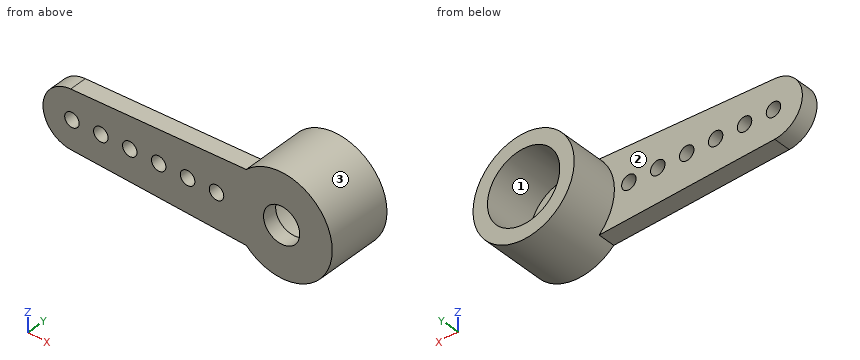
from build123d import *

# Parameters (mm, degrees)
SKETCH_1_R          = 0.5
EXTRUDE_1_DEPTH     = 1.2
SKETCH_1_3_R        = 3.5
SKETCH_1_3_R_2      = 2.5
EXTRUDE_2_DEPTH     = 4.5
SKETCH_1_4_R        = 2.5
EXTRUDE_3_DEPTH     = 1
SKETCH_3_R          = 1.25
CUT_EXTRUDE_1_DEPTH = 1


with BuildPart() as part:
    # 草图1 → 凸台-拉伸1 (new body)
    with BuildSketch(Plane(origin=(0, 0, 0), x_dir=(1, 0, 0), z_dir=(0, 1, 0))):
        with BuildLine():
            Line((4.682566803, 2.501585477), (-7.452442074, 1.998282013))
            ThreePointArc((-7.452442074, 1.998282013), (-9.369562674, 0), (-7.452442074, -1.998282013))
            Line((-7.452442074, -1.998282013), (4.682566803, -2.501585477))
            ThreePointArc((4.682566803, -2.501585477), (3.630437326, 0), (4.682566803, 2.501585477))
        make_face()
        with Locations((-7.369562674, 0)):
            Circle(SKETCH_1_R, mode=Mode.SUBTRACT)
        with Locations((-5.369562674, 0)):
            Circle(SKETCH_1_R, mode=Mode.SUBTRACT)
        with Locations((-3.369562674, 0)):
            Circle(SKETCH_1_R, mode=Mode.SUBTRACT)
        with Locations((-1.369562674, 0)):
            Circle(SKETCH_1_R, mode=Mode.SUBTRACT)
        with Locations((0.630437326, 0)):
            Circle(SKETCH_1_R, mode=Mode.SUBTRACT)
        with Locations((2.630437326, 0)):
            Circle(SKETCH_1_R, mode=Mode.SUBTRACT)
    extrude(amount=EXTRUDE_1_DEPTH)

    # 草图1<3> → 凸台-拉伸2 (add)
    with BuildSketch(Plane(origin=(0, 0, 0), x_dir=(1, 0, 0), z_dir=(0, 1, 0))):
        with Locations((7.130437326, 0)):
            Circle(SKETCH_1_3_R)
        with Locations((7.130437326, 0)):
            Circle(SKETCH_1_3_R_2, mode=Mode.SUBTRACT)
    extrude(amount=EXTRUDE_2_DEPTH)

    # 草图1<4> → 凸台-拉伸3 (add)
    with BuildSketch(Plane(origin=(0, 0, 0), x_dir=(1, 0, 0), z_dir=(0, 1, 0))):
        with Locations((7.130437326, 0)):
            Circle(SKETCH_1_4_R)
    extrude(amount=EXTRUDE_3_DEPTH)

    # 草图3 → 切除-拉伸1 (cut)
    with BuildSketch(Plane(origin=(0, 0, 0), x_dir=(1, 0, 0), z_dir=(0, 1, 0))):
        with Locations((7.130437326, 0)):
            Circle(SKETCH_3_R)
    extrude(amount=CUT_EXTRUDE_1_DEPTH, mode=Mode.SUBTRACT)


solid = part.part
The listing builds one solid part. Answer for the finished solid, in the listing's coordinates (mm). Face numbers are marked on the shaded views. Give positions to 0.01 mm unless a question says otherwise; leave off trailing zeros. Loops run counter-clockwise (first coordinate to the right, second up) from the corner with the lowest first, then second, coordinate; pieces in that order, holes last.
Item 1: Each of these flat-tipped pins is pushed along its axis until it touches: pin 1 Ø1.5 at (y, z) = (0.5, 2) entering from +X; pin 2 Ø4 at (x, z) = (-4, 0) entering from +Y; pin 3 Ø2.5 at (x, z) = (7.5, -1) entering from +Y. Where does it stop, or does it pass through?
Derived:
pin 1: stops at x = 10.4
pin 2: stops at y = 1.2
pin 3: stops at y = 1
Item 2: A cutting plane is placed at D-D (z = 1.5). Give the vertices of the cut face in (x, y), then the cut area to 3 significant figures.
Derived:
outline: (-8.69, 0) - (10.29, 0) - (10.29, 4.5) - (9.13, 4.5) - (9.13, 1) - (5.13, 1) - (5.13, 4.5) - (3.97, 4.5) - (3.97, 1.2) - (-8.69, 1.2) - close
area: 29.7 mm2
Item 3: Find the intervals of material crossed by line 1 along Y through (x, z) = (-0.75, -0.5); line 2 along X through (y, z) = (3.95, 1.75); line 3 along Z through (x, y) = (9.25, 3.05), in increasing order.
Derived:
line 1: y = 0 to 1.2
line 2: x = 4.1 to 5.35, 8.92 to 10.16
line 3: z = -2.79 to -1.33, 1.33 to 2.79
Item 4: A cutting plane is placed at C-C (y = 3.35). Give the vertices of the cut face in (x, z), then the cut area to 3 significant figures.
Derived:
outline: circle Ø7 at (7.13, 0); hole circle Ø5 at (7.13, 0)
area: 18.8 mm2
Item 5: Determine the mould class of the marked faces 1, 2 and 3 for opening direction X: +X half, -X half, draft (parallel to the pull), parting line (faces both ways), or undercut.
Derived:
face 1: undercut
face 2: draft
face 3: parting line
Item 6: A cutting plane is placed at B-B (z = 0). Give the number of separate pieces and of enclosed holes in the cut face, then the cut area to 3 significant figures.
Derived:
separate pieces: 8
enclosed holes: 0
area: 19.9 mm2
Item 7: A cutting plane is placed at A-A (x = 7). Give the vertices of the cut face in (y, z).
Derived:
outline: (0, -3.5) - (4.5, -3.5) - (4.5, -2.5) - (1, -2.5) - (1, -1.24) - (0, -1.24) - close; (0, 1.24) - (1, 1.24) - (1, 2.5) - (4.5, 2.5) - (4.5, 3.5) - (0, 3.5) - close
